from build123d import *
from OCP.BRepFilletAPI import BRepFilletAPI_MakeChamfer

# Parameters (mm, degrees)
SKETCH_1_W               = 41
SKETCH_1_H               = 60
EXTRUDE_1_DEPTH          = 3
SKETCH_2_W               = 41
SKETCH_2_H               = 60
SKETCH_2_W_2             = 38
SKETCH_2_H_2             = 57
EXTRUDE_1_2_DEPTH        = 17
SKETCH_3_W               = 27
SKETCH_3_H               = 3.030341357
CUT_EXTRUDE_1_DEPTH      = 17
SKETCH_4_R               = 2.5
EXTRUDE_2_DEPTH          = 17
CUT_EXTRUDE_2_DEPTH      = 42.475896615
CUT_EXTRUDE_2_DEPTH_BACK = 42.475896615
SKETCH_5_R               = 1.5
SKETCH_9_W               = 41
SKETCH_9_H               = 3
CUT_EXTRUDE_3_DEPTH      = 67.484960705
SKETCH_10_W              = 41
SKETCH_10_H              = 60
EXTRUDE_4_DEPTH          = 2
SKETCH_11_W              = 6
SKETCH_11_H              = 3.013062302
CUT_EXTRUDE_4_DEPTH      = 1
SKETCH_12_W              = 14
SKETCH_12_H              = 6
EXTRUDE_6_DEPTH          = 5
FILLET_2_R               = 1
FILLET_3_R               = 1
FILLET_4_R               = 2
CHAMFER_2_SIZE           = 1
CHAMFER_2_SIZE2          = 1.732050808


with BuildPart() as part:
    # Эскиз1 → Extrude 1 (new body)
    with BuildSketch(Plane(origin=(0, 0, 0), x_dir=(1, 0, 0), z_dir=(0, 1, 0))):
        Rectangle(SKETCH_1_W, SKETCH_1_H)
    extrude(amount=EXTRUDE_1_DEPTH)

    # Эскиз2 → Extrude 1 2 (add)
    with BuildSketch(Plane(origin=(0, 3, 0), x_dir=(1, 0, 0), z_dir=(0, 1, 0))):
        Rectangle(SKETCH_2_W, SKETCH_2_H)
        Rectangle(SKETCH_2_W_2, SKETCH_2_H_2, mode=Mode.SUBTRACT)
    extrude(amount=EXTRUDE_1_2_DEPTH)

    # Эскиз3 → Вырез-Вытянуть1 (cut)
    with BuildSketch(Plane(origin=(0, 20, 0), x_dir=(1, 0, 0), z_dir=(0, 1, 0))):
        with Locations((0, 29.478101209)):
            Rectangle(SKETCH_3_W, SKETCH_3_H)
    extrude(amount=-CUT_EXTRUDE_1_DEPTH, mode=Mode.SUBTRACT)

    # Эскиз4 → Бобышка-Вытянуть2 (add)
    with BuildSketch(Plane(origin=(0, 3, 0), x_dir=(1, 0, 0), z_dir=(0, 1, 0))):
        with Locations((17, 25)):
            Circle(SKETCH_4_R)
        with Locations((-17, 25)):
            Circle(SKETCH_4_R)
        with Locations((17, -25)):
            Circle(SKETCH_4_R)
        with Locations((-17, -25)):
            Circle(SKETCH_4_R)
    extrude(amount=EXTRUDE_2_DEPTH)

    # Эскиз5 → Вырез-Вытянуть2 (cut, two sides: drawn at the far end of the back side and taken through both)
    with BuildSketch(Plane(origin=(0, 20, 0), x_dir=(1, 0, 0), z_dir=(0, 1, 0)).offset(-CUT_EXTRUDE_2_DEPTH_BACK)):
        with Locations(Location((17, 25, 0), (0, 0, 270))):
            Circle(SKETCH_5_R)
        with Locations(Location((17, -25, 0), (0, 0, 270))):
            Circle(SKETCH_5_R)
        with Locations(Location((-17, -25, 0), (0, 0, 270))):
            Circle(SKETCH_5_R)
        with Locations(Location((-17, 25, 0), (0, 0, 270))):
            Circle(SKETCH_5_R)
    extrude(amount=CUT_EXTRUDE_2_DEPTH + CUT_EXTRUDE_2_DEPTH_BACK, mode=Mode.SUBTRACT)

    # Эскиз9 → Вырез-Вытянуть3 (cut, through all)
    with BuildSketch(Plane(origin=(0, 0, -30), x_dir=(-1, 0, 0), z_dir=(0, 0, -1))):
        with Locations((0, 1.5)):
            Rectangle(SKETCH_9_W, SKETCH_9_H)
    extrude(amount=-CUT_EXTRUDE_3_DEPTH, mode=Mode.SUBTRACT)

    # Эскиз10 → Бобышка-Вытянуть4 (add)
    with BuildSketch(Plane(origin=(0, 20, 0), x_dir=(1, 0, 0), z_dir=(0, 1, 0))):
        Rectangle(SKETCH_10_W, SKETCH_10_H)
    extrude(amount=EXTRUDE_4_DEPTH)

    # Эскиз11 → Вырез-Вытянуть4 (cut)
    with BuildSketch(Plane.XZ.offset(-3)):
        with Locations((0, 29.353335514)):
            Rectangle(SKETCH_11_W, SKETCH_11_H)
    extrude(amount=-CUT_EXTRUDE_4_DEPTH, mode=Mode.SUBTRACT)

    # Эскиз12 → Бобышка-Вытянуть6 (add)
    with BuildSketch(Plane.XZ.offset(-20)):
        with Locations((12, 20.5)):
            Rectangle(SKETCH_12_W, SKETCH_12_H)
    extrude(amount=EXTRUDE_6_DEPTH)

    # Скругление2
    fillet_2_edges = [part.edges().sort_by_distance(p)[0] for p in [
        (12, 15, 17.5),
        (5, 17.5, 17.5),
    ]]
    fillet(fillet_2_edges, radius=FILLET_2_R)

    # Скругление3
    fillet_3_edges = [part.edges().sort_by_distance(p)[0] for p in [
        (0, 4, 28.5),
    ]]
    fillet(fillet_3_edges, radius=FILLET_3_R)

    # Скругление4
    fillet_4_edges = [part.edges().sort_by_distance(p)[0] for p in [
        (20.5, 12.5, 30),
        (-20.5, 12.5, 30),
        (-20.5, 12.5, -30),
        (20.5, 12.5, -30),
    ]]
    fillet(fillet_4_edges, radius=FILLET_4_R)

    # Фаска2: one chamfer whose edges measure the first distance from different faces: ONE call of the kernel's chamfer builder (chamfer() names one face for all edges)
    chamfer_2_edges_1 = [part.edges().sort_by_distance(p)[0] for p in [
        (20.5, 22, 0),
    ]]
    chamfer_2_side_1 = [part.faces().sort_by_distance(p)[0] for p in [
        (20.5, 12.5, 0),
    ]]
    chamfer_2_edges_2 = [part.edges().sort_by_distance(p)[0] for p in [
        (0, 22, 30),
    ]]
    chamfer_2_side_2 = [part.faces().sort_by_distance(p)[0] for p in [
        (0, 12.577474892, 30),
    ]]
    chamfer_2_edges_3 = [part.edges().sort_by_distance(p)[0] for p in [
        (-20.5, 22, 0),
    ]]
    chamfer_2_side_3 = [part.faces().sort_by_distance(p)[0] for p in [
        (-20.5, 12.5, 0),
    ]]
    chamfer_2_edges_4 = [part.edges().sort_by_distance(p)[0] for p in [
        (0, 22, -30),
    ]]
    chamfer_2_side_4 = [part.faces().sort_by_distance(p)[0] for p in [
        (-16, 3.415932687, -30),
    ]]
    chamfer_2_edges_5 = [part.edges().sort_by_distance(p)[0] for p in [
        (-19.914213562, 22, 29.414213562),
    ]]
    chamfer_2_side_5 = [part.faces().sort_by_distance(p)[0] for p in [
        (-19.914213562, 12.5, 29.414213562),
    ]]
    chamfer_2_edges_6 = [part.edges().sort_by_distance(p)[0] for p in [
        (-19.914213562, 22, -29.414213562),
    ]]
    chamfer_2_side_6 = [part.faces().sort_by_distance(p)[0] for p in [
        (-19.914213562, 12.5, -29.414213562),
    ]]
    chamfer_2_edges_7 = [part.edges().sort_by_distance(p)[0] for p in [
        (19.914213562, 22, -29.414213562),
    ]]
    chamfer_2_side_7 = [part.faces().sort_by_distance(p)[0] for p in [
        (19.914213562, 12.5, -29.414213562),
    ]]
    chamfer_2_edges_8 = [part.edges().sort_by_distance(p)[0] for p in [
        (19.914213562, 22, 29.414213562),
    ]]
    chamfer_2_side_8 = [part.faces().sort_by_distance(p)[0] for p in [
        (19.914213562, 12.5, 29.414213562),
    ]]
    chamfer_2 = BRepFilletAPI_MakeChamfer(part.part.solid().wrapped)
    for e in chamfer_2_edges_1:
        chamfer_2.Add(CHAMFER_2_SIZE, CHAMFER_2_SIZE2, e.wrapped, chamfer_2_side_1[0].wrapped)  # the first distance lies on this face
    for e in chamfer_2_edges_2:
        chamfer_2.Add(CHAMFER_2_SIZE, CHAMFER_2_SIZE2, e.wrapped, chamfer_2_side_2[0].wrapped)  # the first distance lies on this face
    for e in chamfer_2_edges_3:
        chamfer_2.Add(CHAMFER_2_SIZE, CHAMFER_2_SIZE2, e.wrapped, chamfer_2_side_3[0].wrapped)  # the first distance lies on this face
    for e in chamfer_2_edges_4:
        chamfer_2.Add(CHAMFER_2_SIZE, CHAMFER_2_SIZE2, e.wrapped, chamfer_2_side_4[0].wrapped)  # the first distance lies on this face
    for e in chamfer_2_edges_5:
        chamfer_2.Add(CHAMFER_2_SIZE, CHAMFER_2_SIZE2, e.wrapped, chamfer_2_side_5[0].wrapped)  # the first distance lies on this face
    for e in chamfer_2_edges_6:
        chamfer_2.Add(CHAMFER_2_SIZE, CHAMFER_2_SIZE2, e.wrapped, chamfer_2_side_6[0].wrapped)  # the first distance lies on this face
    for e in chamfer_2_edges_7:
        chamfer_2.Add(CHAMFER_2_SIZE, CHAMFER_2_SIZE2, e.wrapped, chamfer_2_side_7[0].wrapped)  # the first distance lies on this face
    for e in chamfer_2_edges_8:
        chamfer_2.Add(CHAMFER_2_SIZE, CHAMFER_2_SIZE2, e.wrapped, chamfer_2_side_8[0].wrapped)  # the first distance lies on this face
    add(Compound.cast(chamfer_2.Shape()), mode=Mode.REPLACE)


solid = part.part
Input: part model. Units: mm. Frame: model coordinates. A direction names the side the tool comes from. Give positions to 0.01 mm unless a question says otherwise; leave off trailing zeros. Order: outer loops, then holes, each group sorted by start corner. A loop starts at its lowest first (then second) coordinate and runs counter-clockwise, first axis right, second up. Notation, with made-up numbers: (80.5, -2) -> (103.5, -2) arc R30 ccw to (103.5, 28) -> close; hole circle Ø10 at (22, 3.25). An arc over 180 degrees is marked (long way). Use one line per item in the form item = value.
1) Section C-C, the plane z = 21. Return loops of the section in (x, y), and give its area (3 significant figures).
Response values:
outline = (-20.5, 3) -> (-19, 3) -> (-19, 20) -> (5, 20) -> (5, 15) -> (19, 15) -> (19, 3) -> (20.5, 3) -> (20.5, 21) -> (18.77, 22) -> (-18.77, 22) -> (-20.5, 21) -> close
area = 201 mm^2
2) Reachability of faces 4 (the cylindrical face through (-16.93, 11.38, 23.5)), 5 (the flat face through (-13.5, 12, -29)), 6 (the flat face through (-20.5, 12, 0)) from +Z, -Z, +X, -X, +Y, -Y: full face, straight path, thin tool, end or side. Return the list, or none.
Response values:
face_4 = -Y
face_5 = -Z, -Y
face_6 = +Z, -Z, -X, +Y, -Y
3) Mould query, pull axis X, two halves, no side actions, for faces 1 (the flat face through (-19.62, 21.51, -0.39)), 2 (the flat face through (19, 11, 28)), 3 (the flat face through (-19.5, 3, 6.5)). Classes: pulls with the +X half, pulls with the -X half, needs draft (parallel to the pull), parting line crosses it, or undercut.
Response values:
face_1 = pulls with the -X half
face_2 = undercut
face_3 = needs draft
4) Section B-B, the plane x = -12.5. Return loops of the section in (y, z), and give its area (3 significant figures).
Response values:
outline = (3, 28.5) -> (20, 28.5) -> (20, -30) -> (21, -30) -> (22, -28.27) -> (22, 28.27) -> (21, 30) -> (3, 30) -> close
area = 144 mm^2
5) First-contact query: pin 1 Ø6 at (x, y) = (6.5, 14.5) entering from -Z; pin 2 Ø1.5 at (x, z) = (16.5, 25.5) entering from -Y; pin 3 Ø5.5 at (x, z) = (9, 20) entering from -Y. Flat tips, straight axial feed; report the tip coordinate or a pass-through.
Response values:
pin_1 = 17.5
pin_2 = 20
pin_3 = 15
6) Section A-A, the plane y = 6.5. Return loops of the section in (x, z).
Response values:
outline = (-20.5, -28) arc R2 ccw to (-18.5, -30) -> (-13.5, -30) -> (-13.5, -28.5) -> (-19, -28.5) -> (-19, -26.5) arc R2.5 ccw (long way) to (-19, -23.5) -> (-19, 23.5) arc R2.5 ccw (long way) to (-19, 26.5) -> (-19, 28.5) -> (19, 28.5) -> (19, 26.5) arc R2.5 ccw (long way) to (19, 23.5) -> (19, -23.5) arc R2.5 ccw (long way) to (19, -26.5) -> (19, -28.5) -> (13.5, -28.5) -> (13.5, -30) -> (18.5, -30) arc R2 ccw to (20.5, -28) -> (20.5, 28) arc R2 ccw to (18.5, 30) -> (-18.5, 30) arc R2 ccw to (-20.5, 28) -> close; hole circle Ø3 at (-17, -25); hole circle Ø3 at (-17, 25); hole circle Ø3 at (17, -25); hole circle Ø3 at (17, 25)
7) Line query: probe 1 along Z at (x, y) = (-17, 8.25); probe 2 along Z at (x, y) = (17, 16.75); probe 3 along X at (y, z) = (7.25, -25). Output: solid intervals per line, ascending.
Response values:
probe_1 = -30 to -28.5, -27.5 to -26.5, -23.5 to -22.5, 22.5 to 23.5, 26.5 to 27.5, 28.5 to 30
probe_2 = -30 to -28.5, -27.5 to -26.5, -23.5 to -22.5, 17.5 to 23.5, 26.5 to 27.5, 28.5 to 30
probe_3 = -20.5 to -18.5, -15.5 to -14.5, 14.5 to 15.5, 18.5 to 20.5
